Autodesk Inventor part; units mm, degrees
ref_plane "YZ Plane" through (0, 0, 0) normal (1, 0, 0) x (0, 1, 0)
ref_plane "XZ Plane" through (0, 0, 0) normal (0, 1, 0) x (-1, 0, 0)
ref_plane "XY Plane" through (0, 0, 0) normal (0, 0, 1) x (1, 0, 0)
sketch "Sketch1" plane through (0, 0, 0) normal (0, 1, 0) x (-1, 0, 0)
  line L0 (6, 0) -> (-6, 0)
  line L1 (-6, 0) -> (-6, -12)
  line L2 (-6, -12) -> (6, -12)
  line L3 (6, -12) -> (6, 0)
  point P0 (0, 0)
  point P1 (0, 0)
  dimension "d0" = 12
  dimension "d1" = 12
extrude "Extrusion1" add sketch "Sketch1" along normal blind 6
sketch "Sketch2" plane through (0, 6, 0) normal (0, 1, 0) x (1, 0, 0)
  line L0 (6, 12) -> (-6, 12)
  line L1 (-6, 0) -> (6, 0)
  point P0 (0, 0)
  point P1 (0, 9)
  point P2 (0, 0)
  dimension "d4" = 3
hole "Hole1" at (0, 6, -9) direction (0, -1, 0) diameter 4.6 depth 5
fillet "Fillet1" radius 4 2 edges at (-6, 3, -12) (6, 3, -12)
sketch "Sketch3" plane through (-6, 0, 0) normal (0, 0, 1) x (1, 0, 0)
  line L0 (0.5, 2.8) -> (11.5, 2.8)
  line L1 (11.5, 2.8) -> (11.5, 3.2)
  line L2 (11.5, 3.2) -> (0.5, 3.2)
  line L3 (0.5, 3.2) -> (0.5, 2.8)
  line L4 (0, 0) -> (12, 0)
  line L5 (0, 0) -> (0, 6)
  point P0 (6, 0)
  point P1 (6, 2.8)
  point P2 (6, 0)
  point P3 (0.5, 3)
  point P4 (0, 3)
  dimension "d13" = 0.4
  dimension "d14" = 11
extrude "Extrusion2" cut sketch "Sketch3" against normal blind 6
properties part number "AUfsatz" material "ABS Plastic"
Work out the finished part from the listing and answer in its coordinate system (mm). A direction names the side the tool comes from. Give positions to 0.01 mm unless a question says otherwise; leave off trailing zeros. Loops run counter-clockwise (first coordinate to the right, second up) from the corner with the lowest first, then second, coordinate; pieces in that order, holes last. Notation, with made-up numbers: (-33, 41) -> (-25, 41) arc R28 cw to (-25, 78) -> close; hole circle Ø5 at (0, 83.5). An arc over 180 degrees is marked (long way). Use a Markdown table: item, result. Add a question column.
1) Consider line 1 along Y through (x, z) = (-1.25, -3.5); line 2 along Z through (x, y) = (0, 3.9); line 3 along Z through (x, y) = (0, 3). Determine where each line is inside the solid, lowest interval first.
2) This flat-tipped pin is pushed along its axis until it touches: P1, Ø3.5, axis at x = 0.5, z = -9, coming from the +Y side. Where does it stop, or does it pass through?
3) The part is cut by section C-C, the plane x = 0. Determine the outline of the cut face in (y, z).
4) Which of the six approach directions +Z, -Z, +X, -X, +Y, -Y give full straight-line access (tool end or side, diameter ignored) to faces 4 (the flat face through (6, 3, -4)), 5 (the flat face through (0, 1, -9)), 6 (the flat face through (0, 3.2, -3))?
5) The part is cut by section D-D, the plane z = -9. Determine the outline of the cut face in (x, y).
6) For a pull along Y with two mould halves and no side action, classify faces 1 (the flat face through (0, 2.8, -3)), 2 (the flat face through (-6, 3, -4)), 3 (the flat face through (0, 0, -6)) as +Y half, -Y half, draft (parallel to the pull), parting line (faces both ways), or undercut.
7) The part is cut by section A-A, the plane y = 1.95. Determine the outline of the cut face in (x, z).
8) The part is cut by section B-B, the plane z = -3.75. Determine the outline of the cut face in (x, y).
Reported:
| question | item | result |
|---|---|---|
| 1 | line 1 | y = 0 to 2.8, 3.2 to 6 |
| 1 | line 2 | z = -12 to -11.3, -6.7 to 0 |
| 1 | line 3 | z = -12 to -11.3, -6.7 to -6 |
| 2 | P1 | stops at y = 1 |
| 3 | outline | (0, -12) -> (6, -12) -> (6, -11.3) -> (1, -11.3) -> (1, -6.7) -> (6, -6.7) -> (6, 0) -> (3.2, 0) -> (3.2, -6) -> (2.8, -6) -> (2.8, 0) -> (0, 0) -> close |
| 4 | face 4 | +Z, -Z, +X, +Y, -Y |
| 4 | face 5 | +Y |
| 4 | face 6 | +Z |
| 5 | outline | (-5.87, 0) -> (5.87, 0) -> (5.87, 6) -> (2.3, 6) -> (2.3, 1) -> (-2.3, 1) -> (-2.3, 6) -> (-5.87, 6) -> close |
| 6 | face 1 | undercut |
| 6 | face 2 | draft |
| 6 | face 3 | -Y half |
| 7 | outline | (-6, -8) arc R4 ccw to (-2, -12) -> (2, -12) arc R4 ccw to (6, -8) -> (6, 0) -> (-6, 0) -> close; hole circle Ø4.6 at (0, -9) |
| 8 | outline | (-6, 0) -> (6, 0) -> (6, 6) -> (-6, 6) -> close; hole (-5.5, 2.8) -> (5.5, 2.8) -> (5.5, 3.2) -> (-5.5, 3.2) -> close |
